from build123d import *

# Parameters (mm, degrees)
SKETCH1_R           = 2.7
BOSS_EXTRUDE1_DEPTH = 3
SKETCH2_R           = 1.696293742
BOSS_EXTRUDE2_DEPTH = 15.7
CUT_EXTRUDE1_DEPTH  = 2


with BuildPart() as part:
    # Sketch1 → Boss-Extrude1 (new body)
    with BuildSketch(Plane(origin=(0, 0, 0), x_dir=(1, 0, 0), z_dir=(0, 1, 0))):
        with Locations((184.714490272, -125.24429514)):
            Circle(SKETCH1_R)
    extrude(amount=-BOSS_EXTRUDE1_DEPTH)

    # Sketch2 → Boss-Extrude2 (add)
    with BuildSketch(Plane.XZ.offset(3)):
        with Locations((184.714490272, 125.24429514)):
            Circle(SKETCH2_R)
    extrude(amount=BOSS_EXTRUDE2_DEPTH)

    # Sketch3 → Cut-Extrude1 (cut)
    with BuildSketch(Plane(origin=(0, 0, 0), x_dir=(1, 0, 0), z_dir=(0, 1, 0))):
        Polygon((184.714490272, -123.800919467), (183.464490272, -124.522607304), (183.464490272, -125.965982977), (184.714490272, -126.687670813), (185.964490272, -125.965982977), (185.964490272, -124.522607304), align=None)
    extrude(amount=-CUT_EXTRUDE1_DEPTH, mode=Mode.SUBTRACT)


solid = part.part
Here's how the part is built. I have some questions about the finished solid (model axes, mm). A direction names the side the tool comes from. Coordinates: 2 decimals unless noted, no trailing zeros. Write each loop counter-clockwise with the first axis right and the second up, starting at its lowest first coordinate (ties: lowest second). Pieces come first, ordered by that corner, then holes.
Item 1: I want a section at D-D on z = 122.9. Write out the boundary of the cut face in (x, y).
Item 2: I want a section at C-C on y = -3.5. Write out the boundary of the cut face in (x, z), and give its area (3 significant figures).
Item 3: If I drill on line 1 (Y direction, x = 185.1, z = 124.4); line 2 (Y direction, x = 185, z = 123.5); line 3 (X direction, y = -12.5, z = 124.1), over which ranges is the centre line in solid material (lowest first)?
Item 4: On a 3-axis mill with a long thin cutter (end or side, diameter ignored), from which of +Z, -Z, +X, -X, +Y, -Y can I reach the whole of each face in a straight line? I mean faces 1 (the flat face through (184.08, -0.99, 126.32)), 2 (the flat face through (183, -3, 126)), 3 (the flat face through (184, 0, 124)). Say none if no direction works.
Item 5: Will these pins go through, and if not, where does the flat tip stop? pin 1 (1.2 mm diameter, centred on y = -1.5, z = 125.5, fed in from +X); pin 2 (1 mm diameter, centred on y = -12, z = 124, fed in from -X).
Item 6: I want a section at A-A on x = 185.1. Write out the boundary of the cut face in (y, z).
Item 7: If we mould it in two halves opening along Z, with no side actions, what happens to faces 4 (the flat face through (184.098, -0.986, 124.157)), 5 (the flat face through (185, -18.7, 125)), 6 (the cylindrical face through (183.37, -10.74, 124.21))? For each: +Z half, -Z half, draft (parallel to the pull), parting line (faces both ways), or undercut.
Item 8: I want a section at B-B on z = 124.25. Write out the boundary of the cut face in (x, y), and give its area (3 significant figures).
Findings below:
1. outline: (183.37, -3) - (186.05, -3) - (186.05, 0) - (183.37, 0) - close
2. outline: circle Ø3.39 at (184.71, 125.24)
2. area: 9.04 mm2
3. line 1: y = -18.7 to -2
3. line 2: y = -3 to 0
3. line 3: x = 183.46 to 185.97
4. face 1: +Y
4. face 2: -Y
4. face 3: +Z, -Z, +X, -X, +Y
5. pin 1: stops at x = 187.41
5. pin 2: stops at x = 183.19
6. outline: (-18.7, 123.59) - (-3, 123.59) - (-3, 122.57) - (0, 122.57) - (0, 124.02) - (-2, 124.02) - (-2, 126.47) - (0, 126.47) - (0, 127.92) - (-3, 127.92) - (-3, 126.9) - (-18.7, 126.9) - close
7. face 4: undercut
7. face 5: draft
7. face 6: parting line
8. outline: (182.2, -3) - (183.34, -3) - (183.34, -18.7) - (186.09, -18.7) - (186.09, -3) - (187.22, -3) - (187.22, 0) - (185.49, 0) - (185.49, -2) - (183.94, -2) - (183.94, 0) - (182.2, 0) - close
8. area: 55.1 mm2
